Autodesk Fusion 360 part; units mm, degrees
sketch "Sketch1" plane through (0, 0, 0) normal (0, 1, 0) x (1, 0, 0)
  line L0 (-46.4072, 33.7716) -> (-20.4072, 33.7716)
  line L1 (-20.4072, 33.7716) -> (-20.4072, -17.2284)
  line L2 (-20.4072, -17.2284) -> (-46.4072, -17.2284)
  line L3 (-46.4072, -17.2284) -> (-46.4072, 33.7716)
  line L4 (-46.4072, -17.2284) -> (-28.4072, -17.2284)
  line L5 (-28.4072, -17.2284) -> (-28.4072, 27.7716)
  line L6 (-28.4072, 27.7716) -> (-46.4072, 27.7716)
  line L7 (-46.4072, 27.7716) -> (-46.4072, -17.2284)
  line L8 (-28.4072, -17.2284) -> (-12.9072, -17.2284)
  line L9 (-12.9072, -17.2284) -> (-12.9072, 11.7716)
  line L10 (-12.9072, 11.7716) -> (-28.4072, 11.7716)
  line L11 (-28.4072, 11.7716) -> (-28.4072, -17.2284)
  circle A0 centre (-28.4072, 5.2716) radius 18.75
  circle A1 centre (-28.4072, 5.2716) radius 11.5
  line L12 (-48, 35) -> (-48, -19)
  line L13 (-48, -19) -> (-8, -19)
  line L14 (-8, -19) -> (-8, 35)
  line L15 (-8, 35) -> (-48, 35)
  line L16 (-12.9072, -17.2284) -> (-8, -17.2284)
  line L17 (-46.4072, -17.2284) -> (-48, -17.2284)
  line L18 (-46.4072, -17.2284) -> (-46.4072, -19)
  line L19 (-20.4072, -17.2284) -> (-20.4072, -19)
  line L20 (-46.4072, 24.796) -> (-40, 24.796)
  line L21 (-40, 24.796) -> (-40, 27.7716)
  line L22 (-40, 24.796) -> (-37.9936, 21.3857)
  line L23 (-40, 27.7716) -> (-36.6659, 22.1048)
  dimension "d1" = 26
  dimension "d2" = 51
  dimension "d3" = 45
  dimension "d4" = 18
  dimension "d5" = 15.5
  dimension "d6" = 29
  dimension "d7" = 37.5
  dimension "d8" = 23
extrude "Extrude1" add sketch "Sketch1" along normal blind 2 makes body 1
extrude "Extrude2" add sketch "Sketch1" along normal blind 18 separate body contours L0 L1 L3 L7 L9 A0 L12 L14 L15 L16 L17 | L1 L9 L10 A0 A1 | L1 L10 A1 | L3 L7 A0 | L1 L10 A1 | L1 L9 L10 A0 A1 | L1 L8 L9 A0 | L8 L13 L14 L16 L19 | L12 L13 L17 L18 makes body 2
extrude "Extrude3" add sketch "Sketch1" along normal blind 2 separate body contours L0 L1 L3 L7 L9 A0 L12 L14 L15 L16 L17 | L0 L1 L3 L5 L6 A0 | L1 L9 L10 A0 A1 | L1 L5 A0 A1 | L3 L7 A0 L20 L22 | A0 L21 L22 L23 | L5 L6 A0 L23 | L1 L10 A1 | L1 L5 L10 A1 | L3 L5 L7 L11 A0 A1 | L3 L7 A0 | L1 L10 A1 | L1 L5 L10 L11 A1 | L1 L9 L10 A0 A1 | L5 L11 A1 | L1 L8 L9 A0 | L2 L3 L4 L5 L7 L11 A0 | L1 L5 L11 A0 A1 | L8 L13 L14 L16 L19 | L1 L2 L5 L8 L11 A0 | L12 L13 L17 L18 | L2 L4 L8 L13 L18 L19 makes body 3
extrude "Extrude4" add sketch "Sketch1" along normal blind 8 separate body contours L0 L1 L3 L7 L9 A0 L12 L14 L15 L16 L17 | L0 L1 L3 L5 L6 A0 | L1 L9 L10 A0 A1 | L1 L5 A0 A1 | L1 L10 A1 | L1 L5 L10 A1 | L3 L7 A0 | L8 L13 L14 L16 L19 | L12 L13 L17 L18 picked at (-14.7995, 12.9513) picked at (-19.8853, 12.3809) makes body 4
extrude "Extrude5" add sketch "Sketch1" along normal blind 2 separate body contours L0 L1 L3 L7 L9 A0 L12 L14 L15 L16 L17 | L0 L1 L3 L5 L6 A0 | L1 L9 L10 A0 A1 | L1 L5 A0 A1 | L3 L7 A0 L20 L22 | A0 L21 L22 L23 | L5 L6 A0 L23 | L1 L10 A1 | L1 L5 L10 A1 | L3 L5 L7 L11 A0 A1 | L3 L7 A0 | L1 L10 A1 | L1 L5 L10 L11 A1 | L1 L9 L10 A0 A1 | L5 L11 A1 | L1 L8 L9 A0 | L2 L3 L4 L5 L7 L11 A0 | L1 L5 L11 A0 A1 | L8 L13 L14 L16 L19 | L1 L2 L5 L8 L11 A0 | L12 L13 L17 L18 | L2 L4 L8 L13 L18 L19 makes body 5
extrude "Extrude6" add sketch "Sketch1" along normal blind 3 separate body contours L0 L1 L3 L7 L9 A0 L12 L14 L15 L16 L17 | L0 L1 L3 L5 L6 A0 | L3 L7 A0 L20 L22 | L5 L6 A0 L23 | L1 L10 A1 | L1 L5 L10 A1 | L1 L10 A1 | L1 L5 L10 L11 A1 | L5 L11 A1 | L1 L8 L9 A0 | L2 L3 L4 L5 L7 L11 A0 | L8 L13 L14 L16 L19 | L1 L2 L5 L8 L11 A0 | L12 L13 L17 L18 | L2 L4 L8 L13 L18 L19 makes body 6 at (-32, 3, -32.5905) makes body 7 at (-31.134, 0, -9.3605)
move_body "Move1" bodies 2 to x (1, 0, 0) y (0, 1, 0) z (0, 0, 1) at (0, 2, 0)
move_body "Move2" bodies 3 to x (1, 0, 0) y (0, 1, 0) z (0, 0, 1) at (0, 20, 0)
move_body "Move3" bodies 4 to x (1, 0, 0) y (0, 1, 0) z (0, 0, 1) at (0, 22, 0)
move_body "Move4" bodies 5 to x (1, 0, 0) y (0, 1, 0) z (0, 0, 1) at (0, 30, 0)
move_body "Move5" bodies 6 to x (1, 0, 0) y (0, 1, 0) z (0, 0, 1) at (0, 32, 0)
move_body "Move6" bodies 7 to x (1, 0, 0) y (0, 1, 0) z (0, 0, 1) at (0, 32, 0)
combine "Combine1" operation add target body 1 tool bodies 7 6 2 4 3 5
Design review of the part built by this model. Coordinates are the model's own, in mm. A direction names the side the tool comes from. Round coordinates to 2 decimals unless told otherwise and drop trailing zeros. Write each loop counter-clockwise with the first axis right and the second up, starting at its lowest first coordinate (ties: lowest second). Pieces come first, ordered by that corner, then holes. Notation, with made-up numbers: (66.25, 21.5) - (99.25, 21.5) arc R34 cw to (99.25, 60.5) - close; hole circle Ø4 at (41, 9). An arc over 180 degrees is marked (long way). Return JSON: item names as keys, results as strings. Group by question number.
Item 1: We need section C-C on z = -8. Write out the cut boundary in (x, y).
Item 2: We need section D-D on x = -16. Write out the cut boundary in (y, z).
Item 3: The part is to be moulded in two halves that separate along Y. For faces 1 (the face through (-43, 32, -24.796)), 2 (the face through (-17, 26, 17.228)), 3 (the face through (-33, 32, 6)), 4 (the face through (-12.907, 26, 3)), say which applies: pulls with the +Y half, pulls with the -Y half, needs draft (parallel to the pull), parting line crosses it, or undercut.
Item 4: We need section A-A on y = 6.5. Write out the cut boundary in (x, z).
Item 5: For probe 1 along Y at (x, z) = (-31, -18.5); probe 2 along Y at (x, z) = (-38, -2); probe 3 along X at (y, z) = (17.5, 17), list the stretches that pass through material, from the lowest coordinate up. Write a range as [from, to].
Item 6: Insertion check: P1, Ø6, axis at x = -40.5, y = 11, coming from the +Z side. The pin has a flat end and moves straight along its axis. Give the tip position at first contact, or say it passes through.
Item 7: Machinability: for faces 5 (the face through (-43, 21, -24.796)), 6 (the face through (-28.407, 26, -20)), 7 (the face through (-21, 26, -11.772)), which of the approach directions +Z, -Z, +X, -X, +Y, -Y give a long, thin tool a straight path to every point of the face, cutting with its end or side? Answer none if there is none.
Item 8: We need section B-B on x = -43. Write out the cut boundary in (y, z), and give its area (3 significant figures).
Model answer:
{
 "1": {"outline": "(-48, 0) - (-8, 0) - (-8, 35) - (-9.86, 35) - (-9.86, 32) - (-17.24, 32) - (-17.24, 35) - (-39.58, 35) - (-39.58, 32) - (-46.96, 32) - (-46.96, 35) - (-48, 35) - close; hole (-46.41, 2) - (-20.41, 2) - (-20.41, 20) - (-46.41, 20) - close; hole (-46.41, 22) - (-12.91, 22) - (-12.91, 30) - (-46.41, 30) - close"},
 "2": {"outline": "(0, -35) - (35, -35) - (35, -19.33) - (32, -19.33) - (32, 8.79) - (35, 8.79) - (35, 19) - (0, 19) - close; hole (22, -11.77) - (30, -11.77) - (30, 17.23) - (22, 17.23) - close"},
 "3": {"face 1": "needs draft", "face 2": "undercut", "face 3": "pulls with the +Y half", "face 4": "undercut"},
 "4": {"outline": "(-48, -35) - (-8, -35) - (-8, 19) - (-20.41, 19) - (-20.41, -33.77) - (-46.41, -33.77) - (-46.41, 19) - (-48, 19) - close"},
 "5": {"probe 1": "y = [0, 2], [20, 22], [30, 32]", "probe 2": "y = [0, 2], [20, 22], [30, 35]", "probe 3": "x = [-48, -46.41], [-20.41, -8]"},
 "6": {"P1": "stops at z = -33.77"},
 "7": {"face 5": "+Y", "face 6": "+Z", "face 7": "none"},
 "8": {"outline": "(0, -35) - (35, -35) - (35, -27.77) - (20, -27.77) - (20, -33.77) - (2, -33.77) - (2, 19) - (0, 19) - close; (20, -24.8) - (22, -24.8) - (22, 19) - (20, 19) - close; (30, -24.8) - (35, -24.8) - (35, -17.04) - (32, -17.04) - (32, 6.5) - (35, 6.5) - (35, 19) - (30, 19) - close", "area": "474 mm²"}
}
